The listing builds one solid part. Answer for the finished solid, in the listing's coordinates (mm). A direction names the side the tool comes from. Coordinates: 2 decimals unless noted, no trailing zeros. Write each loop counter-clockwise with the first axis right and the second up, starting at its lowest first coordinate (ties: lowest second). Pieces come first, ordered by that corner, then holes.
from build123d import *

# Parameters (mm, degrees)
SKETCH1_W               = 50
SKETCH1_H               = 15
BOSS_EXTRUDE1_DEPTH     = 35
SKETCH3_W               = 60
SKETCH3_H               = 70
BOSS_EXTRUDE2_DEPTH     = 5
SKETCH2_R               = 2.5
CUT_EXTRUDE1_DEPTH      = 1
CUT_EXTRUDE1_DEPTH_BACK = 10
FILLET1_R               = 2


with BuildPart() as part:
    # Sketch1 → Boss-Extrude1 (new body, symmetric)
    with BuildSketch(Plane.XY):
        Rectangle(SKETCH1_W, SKETCH1_H)
    extrude(amount=BOSS_EXTRUDE1_DEPTH, both=True)

    # Sketch3 → Boss-Extrude2 (add)
    with BuildSketch(Plane(origin=(0, 7.5, 0), x_dir=(1, 0, 0), z_dir=(0, 1, 0))):
        Rectangle(SKETCH3_W, SKETCH3_H)
    extrude(amount=BOSS_EXTRUDE2_DEPTH)

    # Sketch2 → Cut-Extrude1 (cut, two sides)
    with BuildSketch(Plane(origin=(0, 12.5, 0), x_dir=(1, 0, 0), z_dir=(0, 1, 0))) as cut_extrude1_sk:
        Circle(SKETCH2_R)
    extrude(amount=CUT_EXTRUDE1_DEPTH, mode=Mode.SUBTRACT)
    extrude(cut_extrude1_sk.sketch, amount=-CUT_EXTRUDE1_DEPTH_BACK, mode=Mode.SUBTRACT)

    # Fillet1
    fillet1_edges = [part.edges().sort_by_distance(p)[0] for p in [
        (-30, 12.5, 0),
        (30, 12.5, 0),
    ]]
    fillet(fillet1_edges, radius=FILLET1_R)


solid = part.part
1. Flat-ended cylindrical pins translate along their axes: P1, Ø7.5, axis at y = -3, z = -1.5, coming from the -X side; P2, Ø1.5, axis at x = -27.5, z = 12.5, coming from the -Y side; P3, Ø4.5, axis at y = -1, z = -3.5, coming from the +X side. Find the tip coordinate at first contact, or state that the pin passes through.
Results found:
P1: stops at x = -25
P2: stops at y = 7.5
P3: stops at x = 25
2. Section B-B on z = 14.5 is taken. Give the vertices of the cut face in (x, y), then the cut area to 3 significant figures.
Results found:
outline: (-30, 7.5) - (-25, 7.5) - (-25, -7.5) - (25, -7.5) - (25, 7.5) - (30, 7.5) - (30, 10.5) arc R2 ccw to (28, 12.5) - (-28, 12.5) arc R2 ccw to (-30, 10.5) - close
area: 1,050 mm2
3. For a pull along X with two mould halves and no side action, classify faces 1 (the cylindrical face through (-0.54, 7.57, 2.44)), 2 (the cylindrical face through (-29.43, 11.9, -0.49)), 3 (the flat face through (0, 2, 35)), 4 (the flat face through (0, 2.5, 0)) as pulls with the +X half, pulls with the -X half, needs draft (parallel to the pull), parting line crosses it, or undercut.
Results found:
face 1: undercut
face 2: pulls with the -X half
face 3: needs draft
face 4: undercut
4. A tool of negligible diameter and unlimited length cuts with its end or side. For faces 5 (the flat face through (0, 2, -35)), 6 (the flat face through (-28, 7.5, 0)), 7 (the flat face through (25, 0, 0)), from which of +Z, -Z, +X, -X, +Y, -Y can it reach the whole face along a straight path? Write none if from no direction.
Results found:
face 5: -Z, +X, -X, +Y, -Y
face 6: +Z, -Z, -X, -Y
face 7: +Z, -Z, +X, -Y
5. Find the intervals of material crossed by L1, parallel to Z at x = 0, y = 7.75; L2, parallel to X at y = 6.25, z = 0; L3, parallel to X at y = 8.5, z = 0, in increasing order.
Results found:
L1: z = -35 to -2.5, 2.5 to 35
L2: x = -25 to -2.5, 2.5 to 25
L3: x = -30 to -2.5, 2.5 to 30
6. Section A-A on x = 0 is taken. Give the vertices of the cut face in (y, z), then the cut area to 3 significant figures.
Results found:
outline: (-7.5, -35) - (12.5, -35) - (12.5, -2.5) - (2.5, -2.5) - (2.5, 2.5) - (12.5, 2.5) - (12.5, 35) - (-7.5, 35) - close
area: 1,350 mm2
7. Section D-D on z = 0 is taken. Give the vertices of the cut face in (x, y), then the cut area to 3 significant figures.
Results found:
outline: (-30, 7.5) - (-25, 7.5) - (-25, -7.5) - (25, -7.5) - (25, 7.5) - (30, 7.5) - (30, 10.5) arc R2 ccw to (28, 12.5) - (2.5, 12.5) - (2.5, 2.5) - (-2.5, 2.5) - (-2.5, 12.5) - (-28, 12.5) arc R2 ccw to (-30, 10.5) - close
area: 998 mm2
8. Section C-C on y = -5.25 is taken. Give the vertices of the cut face in (x, z).
Results found:
outline: (-25, -35) - (25, -35) - (25, 35) - (-25, 35) - close
